Design review of the part built by this model. Coordinates are the model's own, in mm. A direction names the side the tool comes from. Give positions to 0.01 mm unless a question says otherwise; leave off trailing zeros. Order: outer loops, then holes, each group sorted by start corner. A loop starts at its lowest first (then second) coordinate and runs counter-clockwise, first axis right, second up. Notation, with made-up numbers: (73, 77.25) - (87, 77.25) arc R13 ccw to (87, 91.25) - close; hole circle Ø2 at (82, -28.75). An arc over 180 degrees is marked (long way). Write each question's results on one line, items separated by ' | '. Start each with the question number.
```python
from build123d import *

# Parameters (mm, degrees)
F0_R      = 20
F1_DEPTH  = 6
F2_R      = 12
F3_DEPTH  = 4.25
F4_R      = 12.75
F5_DEPTH  = 5.5
F6_R      = 12
F7_DEPTH  = 4.25
F8_R      = 20
F9_DEPTH  = 6
F10_R     = 5
F11_DEPTH = 26.001
F12_SIZE2 = 1.6
F12_SIZE  = 6
F13_SIZE2 = 6
F13_SIZE  = 1.5


with BuildPart() as f1:
    # F0 (on Top) → F1 (new body)
    with BuildSketch(Plane.XY):
        Circle(F0_R)
    extrude(amount=F1_DEPTH)

    # F2 (on face) → F3 (join)
    with BuildSketch(Plane.XY.offset(6)):
        Circle(F2_R)
    extrude(amount=F3_DEPTH)

    # F4 (on face) → F5 (join)
    with BuildSketch(Plane.XY.offset(10.25)):
        Circle(F4_R)
    extrude(amount=F5_DEPTH)

    # F6 (on face) → F7 (join)
    with BuildSketch(Plane.XY.offset(15.75)):
        Circle(F6_R)
    extrude(amount=F7_DEPTH)

    # F8 (on face) → F9 (join)
    with BuildSketch(Plane.XY.offset(20)):
        Circle(F8_R)
    extrude(amount=F9_DEPTH)

    # F10 (on face) → F11 (cut, through all)
    with BuildSketch(Plane.XY.offset(26)):
        Circle(F10_R)
    extrude(amount=-F11_DEPTH, mode=Mode.SUBTRACT)

    # F12
    f12_edges = [f1.edges().sort_by_distance(p)[0] for p in [
        (-20, 0, 6),
    ]]
    f12_side = f1.faces().sort_by_distance((-19.434315, 0, 6))[0]
    chamfer(f12_edges, length=F12_SIZE, length2=F12_SIZE2, reference=f12_side)

    # F13
    f13_edges = [f1.edges().sort_by_distance(p)[0] for p in [
        (-20, 0, 20),
    ]]
    f13_side = f1.faces().sort_by_distance((-20, 0, 23))[0]
    chamfer(f13_edges, length=F13_SIZE, length2=F13_SIZE2, reference=f13_side)


solid = f1.part
```
Q1. Machinability: for faces 4 (the cylindrical face through (-4.336, -19.524, 23.718)), 5 (the flat face through (11.3, -4.7, 15.75)), which of the approach directions +Z, -Z, +X, -X, +Y, -Y give a long, thin tool a straight path to every point of the face, cutting with its end or side? Answer none if there is none.
Q2. Insertion check: pin 1 Ø12 at (y, z) = (-11, 21) entering from +X; pin 2 Ø3 at (y, z) = (8, 11) entering from +X; pin 3 Ø2 at (x, z) = (11, 12) entering from -Y. Each pin has a flat end and moves straight along its axis. Give the tip position at first contact, or say it passes through.
Q3. Draft analysis for pull direction Z (two halves, no side actions). For faces 1 (the flat face through (4, -4, 0)), 2 (the conical face through (-3.12, -14.03, 5.9)), 3 (the cylindrical face through (-4.336, -19.524, 2.169)), state which applies: pulls with the +Z half, pulls with the -Z half, needs draft (parallel to the pull), parting line crosses it, or undercut.
Q4. Add section A-A (x = 0). Give the boundary of the cut face in (y, z).
Q5. For line 1 (Y direction, x = 0, z = 12.75); line 2 (Y direction, x = 1.5, z = 12.75); line 3 (Z direction, x = -16.5, y = 9), list the stretches that pass through material, from the lowest coordinate up. Write a range as [from, to].
Q6. Add section C-C (z = 11.5). Give the boundary of the cut face in (x, y), plus the area to 3 significant figures.
Q7. Add section D-D (z = 20.5). Give the boundary of the cut face in (x, y).
Verdict:
1) face 4: +Z, -Z | face 5: none
2) pin 1: stops at x = 19.36 | pin 2: stops at x = 10.97 | pin 3: stops at y = -7.91
3) face 1: pulls with the -Z half | face 2: undercut | face 3: needs draft
4) outline: (-20, 0) - (-5, 0) - (-5, 26) - (-20, 26) - (-20, 21.5) - (-14, 20) - (-12, 20) - (-12, 15.75) - (-12.75, 15.75) - (-12.75, 10.25) - (-12, 10.25) - (-12, 6) - (-14, 6) - (-20, 4.4) - close; (5, 0) - (20, 0) - (20, 4.4) - (14, 6) - (12, 6) - (12, 10.25) - (12.75, 10.25) - (12.75, 15.75) - (12, 15.75) - (12, 20) - (14, 20) - (20, 21.5) - (20, 26) - (5, 26) - close
5) line 1: y = [-12.75, -5], [5, 12.75] | line 2: y = [-12.66, -4.77], [4.77, 12.66] | line 3: z = [0, 4.72], [21.2, 26]
6) outline: circle Ø25.5 at (0, 0); hole circle Ø10 at (0, 0) | area: 432 mm2
7) outline: circle Ø32 at (0, 0); hole circle Ø10 at (0, 0)
